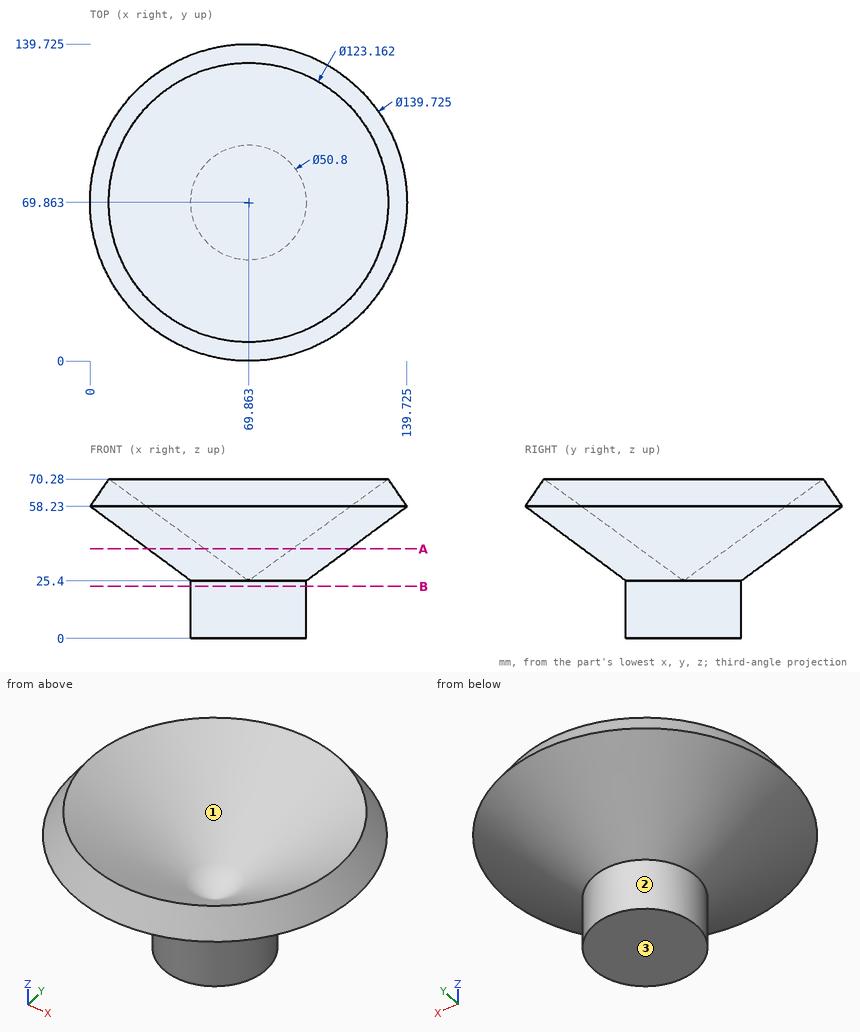
Job drawing, mm, ordinate dimensions from the low corner. One solid piece. Round coordinates to 2 decimals unless told otherwise and drop trailing zeros. Write each loop counter-clockwise with the first axis right and the second up, starting at its lowest first coordinate (ties: lowest second). Pieces come first, ordered by that corner, then holes. Notation, with made-up numbers: (62, 74) -> (118, 74) arc R34 ccw to (118, 111) -> close; hole circle Ø9 at (10.5, 19). An arc over 180 degrees is marked (long way). Answer as CSV lines item,"result".
1. Mould opens along X. For the marked faces 1, 2 and 3 say: +X half, -X half, draft (parallel to the pull), parting line (faces both ways), or undercut.
Resolved:
face 1,"undercut"
face 2,"parting line"
face 3,"draft"
2. Slice it at A-A, the plane z = 39.5. List the corners of the cut face in (x, y) (1 decimal), plus the area to 3 significant figures.
Resolved:
outline,"circle Ø89 at (69.9, 69.9); hole circle Ø38.7 at (69.9, 69.9)"
area,"5,040 mm²"
3. Pin check, flat tips, straight feed: pin 1 Ø1.5 at (x, y) = (84, 105) entering from +Z; pin 2 Ø3 at (y, z) = (95.5, 52) entering from -X; pin 3 Ø3 at (y, z) = (81.5, 28) entering from +X (1 decimal). Stop position of each tip, or through.
Resolved:
pin 1,"z = 53.55"
pin 2,"x = 11.72"
pin 3,"x = 98.6"
4. Slice it at B-B, the plane z = 23. List the corners of the cut face in (x, y).
Resolved:
outline,"circle Ø50.8 at (69.86, 69.86)"
5. Drill centre lines: line 1 (X direction, y = 89.5, z = 54.5) (1 decimal); line 2 (X direction, y = 60.5, z = 39.5) (1 decimal); line 3 (X direction, y = 63.5, z = 4). Where is each one in solid material? Low to high.
Resolved:
line 1,"8.1 to 35.1, 104.6 to 131.6"
line 2,"26.4 to 52.9, 86.8 to 113.4"
line 3,"45.27 to 94.45"
